```python
from build123d import *

# Parameters (mm, degrees)
BOSS_EXTRUDE1_DEPTH = 2.54
BOSS_EXTRUDE2_DEPTH = 2.54
BOSS_EXTRUDE3_DEPTH = 2.54
SKETCH6_W           = 2.54
SKETCH6_H           = 76.2
BOSS_EXTRUDE4_DEPTH = 76.2
CUT_EXTRUDE1_REACH  = 133.982
SKETCH8_W           = 2.54
SKETCH8_H           = 78.74
BOSS_EXTRUDE5_DEPTH = 76.2
CUT_EXTRUDE2_REACH  = 133.982
SKETCH10_W          = 78.74
SKETCH10_H          = 2.54
BOSS_EXTRUDE6_DEPTH = 76.2
CUT_EXTRUDE3_REACH  = 133.982
CUT_EXTRUDE5_DEPTH  = 132.982271537
CUT_EXTRUDE6_DEPTH  = 132.982271537
CUT_EXTRUDE9_DEPTH  = 76.2
BOSS_EXTRUDE7_DEPTH = 7.62
BOSS_EXTRUDE8_DEPTH = 5.08
BOSS_EXTRUDE9_DEPTH = 5.08
SKETCH34_R          = 2
CUT_EXTRUDE11_DEPTH = 12.7
SKETCH35_R          = 2
CUT_EXTRUDE13_DEPTH = 12.7
SKETCH36_R          = 2
CUT_EXTRUDE14_DEPTH = 12.7


with BuildPart() as part:
    # Sketch1 → Boss-Extrude1 (new body)
    with BuildSketch(Plane.XY):
        Polygon((0, 76.2), (0, 0), (76.2, 0), (76.2, 25.4), (25.4, 76.2), align=None)
    extrude(amount=BOSS_EXTRUDE1_DEPTH)

    # Sketch3 → Boss-Extrude2 (add)
    with BuildSketch(Plane.ZY):
        Polygon((0, 76.2), (25.4, 76.2), (76.2, 25.4), (76.2, 0), (0, 0), align=None)
    extrude(amount=BOSS_EXTRUDE2_DEPTH)

    # Sketch5 → Boss-Extrude3 (add)
    with BuildSketch(Plane.XZ):
        Polygon((-2.54, 76.2), (-2.54, 0), (76.2, 0), (76.2, 25.4), (22.86, 76.2), align=None)
    extrude(amount=BOSS_EXTRUDE3_DEPTH)

    # Sketch6 → Boss-Extrude4 (add)
    with BuildSketch(Plane.XY):
        with Locations((3.81, 38.1)):
            Rectangle(SKETCH6_W, SKETCH6_H)
    extrude(amount=BOSS_EXTRUDE4_DEPTH)

    # Sketch7 → Cut-Extrude1 (cut, up to next)
    with BuildSketch(Plane(origin=(0, 0, 0), x_dir=(0, 0, -1), z_dir=(1, 0, 0)), mode=Mode.PRIVATE) as cut_extrude1_sk1:
        Polygon((-25.4, 76.2), (-76.2, 25.4), (-76.2, 76.2), align=None)
    cut_extrude1_tool1 = extrude(cut_extrude1_sk1.sketch, amount=CUT_EXTRUDE1_REACH, mode=Mode.PRIVATE) & part.part
    add(cut_extrude1_tool1.solids().sort_by_distance((0, 59.266667, 59.266667))[0], mode=Mode.SUBTRACT)

    # Sketch8 → Boss-Extrude5 (add)
    with BuildSketch(Plane(origin=(0, 0, 0), x_dir=(0, 0, -1), z_dir=(1, 0, 0))):
        with Locations((-6.35, 36.83)):
            Rectangle(SKETCH8_W, SKETCH8_H)
    extrude(amount=BOSS_EXTRUDE5_DEPTH)

    # Sketch9 → Cut-Extrude2 (cut, up to next)
    with BuildSketch(Plane.XY, mode=Mode.PRIVATE) as cut_extrude2_sk1:
        Polygon((76.2, 25.4), (25.4, 76.2), (76.2, 76.2), align=None)
    cut_extrude2_tool1 = extrude(cut_extrude2_sk1.sketch, amount=CUT_EXTRUDE2_REACH, mode=Mode.PRIVATE) & part.part
    add(cut_extrude2_tool1.solids().sort_by_distance((59.266667, 59.266667, 0))[0], mode=Mode.SUBTRACT)

    # Sketch10 → Boss-Extrude6 (add)
    with BuildSketch(Plane.XY):
        with Locations((36.83, 3.81)):
            Rectangle(SKETCH10_W, SKETCH10_H)
    extrude(amount=BOSS_EXTRUDE6_DEPTH)

    # Sketch11 → Cut-Extrude3 (cut, up to next)
    with BuildSketch(Plane(origin=(0, 0, 0), x_dir=(1, 0, 0), z_dir=(0, 1, 0)), mode=Mode.PRIVATE) as cut_extrude3_sk1:
        Polygon((22.86, -76.2), (76.2, -25.4), (76.2, -76.2), align=None)
    cut_extrude3_tool1 = extrude(cut_extrude3_sk1.sketch, amount=CUT_EXTRUDE3_REACH, mode=Mode.PRIVATE) & part.part
    add(cut_extrude3_tool1.solids().sort_by_distance((58.42, 0, 59.266667))[0], mode=Mode.SUBTRACT)

    # Sketch12 → Cut-Extrude5 (cut, through all)
    with BuildSketch(Plane(origin=(0, 0, 0), x_dir=(0, 0, -1), z_dir=(1, 0, 0))):
        Polygon((-5.08, 5.08), (-5.08, 2.54), (-7.62, 2.54), (-7.62, 0), (-2.54, 0), (-2.54, 5.08), align=None)
    extrude(amount=CUT_EXTRUDE5_DEPTH, mode=Mode.SUBTRACT)

    # Sketch13 → Cut-Extrude6 (cut, through all)
    with BuildSketch(Plane(origin=(0, 0, 0), x_dir=(1, 0, 0), z_dir=(0, 1, 0))):
        Polygon((0, -2.54), (0, -7.62), (2.54, -7.62), (2.54, -5.08), (5.08, -5.08), (5.08, -2.54), align=None)
    extrude(amount=CUT_EXTRUDE6_DEPTH, mode=Mode.SUBTRACT)

    # Sketch15 → Cut-Extrude9 (cut)
    with BuildSketch(Plane.XY.offset(2.54)):
        Polygon((2.54, 5.08), (0, 5.08), (0, 0), (5.08, 0), (5.08, 2.54), (2.54, 2.54), align=None)
    extrude(amount=CUT_EXTRUDE9_DEPTH, mode=Mode.SUBTRACT)


with BuildPart() as cut_extrude9_piece_1:
    # of the separate pieces the step leaves, piece 1, a body of its own (cut_extrude9_pieces)
    add(part.part.solids().sort_by_distance((0, 0, 2.54))[0])



with BuildPart() as cut_extrude9_piece_2:
    # of the separate pieces the step leaves, piece 2, a body of its own (cut_extrude9_pieces)
    add(part.part.solids().sort_by_distance((2.54, 2.54, 76.2))[0])


with BuildPart() as cut_extrude9_piece_1_1:
    add(cut_extrude9_piece_1.part)

    add(cut_extrude9_piece_2.part)  # Boss-Extrude7 merges Cut-Extrude9 piece 2
    # Sketch17 → Boss-Extrude7 (add)
    with BuildSketch(Plane(origin=(0, 0, 0), x_dir=(-1, 0, 0), z_dir=(0, 0, -1))):
        Polygon((-67.219743879, 34.380256121), (-34.380256121, 67.219743879), (-30.788153673, 63.627641431), (-63.627641431, 30.788153673), align=None)
    extrude(amount=-BOSS_EXTRUDE7_DEPTH)

    # Sketch18 → Boss-Extrude8 (add)
    with BuildSketch(Plane(origin=(0, 0, 0), x_dir=(1, 0, 0), z_dir=(0, 1, 0))):
        Polygon((32.056551724, -67.44137931), (67.003448276, -34.15862069), (63.5, -30.48), (28.553103448, -63.762758621), align=None)
    extrude(amount=BOSS_EXTRUDE8_DEPTH)

    # Sketch19 → Boss-Extrude9 (add)
    with BuildSketch(Plane(origin=(0, 0, 0), x_dir=(0, 0, -1), z_dir=(1, 0, 0))):
        Polygon((-32.545001849, 69.054998151), (-67.219743879, 34.380256121), (-63.627641431, 30.788153673), (-28.9528994, 65.462895703), align=None)
    extrude(amount=BOSS_EXTRUDE9_DEPTH)

    # Sketch34 → Cut-Extrude11 (cut, symmetric)
    with BuildSketch(Plane(origin=(0, 0, 0), x_dir=(0, 0, -1), z_dir=(1, 0, 0))):
        with Locations((-15.24, 57.15)):
            Circle(SKETCH34_R)
        with Locations((-15.24, 29.21)):
            Circle(SKETCH34_R)
        with Locations((-31.75, 12.7)):
            Circle(SKETCH34_R)
        with Locations((-57.15, 12.7)):
            Circle(SKETCH34_R)
    extrude(amount=CUT_EXTRUDE11_DEPTH, both=True, mode=Mode.SUBTRACT)

    # Sketch35 → Cut-Extrude13 (cut, symmetric)
    with BuildSketch(Plane(origin=(0, 0, 0), x_dir=(1, 0, 0), z_dir=(0, 1, 0))):
        with Locations(Location((12.7, -57.15, 0), (0, 0, 270))):
            Circle(SKETCH35_R)
        with Locations(Location((12.7, -31.75, 0), (0, 0, 270))):
            Circle(SKETCH35_R)
        with Locations(Location((29.21, -15.24, 0), (0, 0, 270))):
            Circle(SKETCH35_R)
        with Locations(Location((57.15, -15.24, 0), (0, 0, 270))):
            Circle(SKETCH35_R)
    extrude(amount=CUT_EXTRUDE13_DEPTH, both=True, mode=Mode.SUBTRACT)

    # Sketch36 → Cut-Extrude14 (cut, symmetric)
    with BuildSketch(Plane.XY):
        with Locations((57.15, 12.7)):
            Circle(SKETCH36_R)
        with Locations((29.21, 12.7)):
            Circle(SKETCH36_R)
        with Locations((12.7, 29.21)):
            Circle(SKETCH36_R)
        with Locations((12.7, 57.15)):
            Circle(SKETCH36_R)
    extrude(amount=CUT_EXTRUDE14_DEPTH, both=True, mode=Mode.SUBTRACT)


solid = cut_extrude9_piece_1_1.part
```
The listing builds one solid part. Answer for the finished solid, in the listing's coordinates (mm). A direction names the side the tool comes from. Coordinates: 2 decimals unless noted, no trailing zeros. Order: outer loops, then holes, each group sorted by start corner. A loop starts at its lowest first (then second) coordinate and runs counter-clockwise, first axis right, second up. Notation, with made-up numbers: M 39.25,23 L 98.25,23 A26 cw 98.25,39 Z; hole C 79.5,28 d8. An arc over 180 degrees is marked long. Answer as a JSON object with one key per item and string values. Group by question number.
1. Section A-A on z = 24 is taken. Write down the section's boundary in (x, y), then the cut area to 3 significant figures.
2. Straight lines are drawn through the part: line 1 (Y direction, x = 4, z = 15); line 2 (Y direction, x = 43, z = 12); line 3 (Z direction, x = 31.5, y = 33.5). For each, find the intervals that lie inside material, in ascending order.
3. Section B-B on y = 20 is taken. Write down the section's boundary in (x, z).
4. A tool of negligible diameter and unlimited length cuts with its end or side. For faces 5 (the flat face through (32, 33, 7.62)), 6 (the cylindrical face through (11.934, -1.252, 33.597)), 7 (the flat face through (46.27, 1.25, 46.89)), from which of +Z, -Z, +X, -X, +Y, -Y can it reach the whole face along a straight path? Write none if from no direction.
5. Section D-D on z = 57.5 is taken. Write down the section's boundary in (x, y) (3 decimals).
6. Section C-C on x = 60.5 is taken. Write down the section's boundary in (y, z).
7. Determine the mould class of faces 1 (the cylindrical face through (11.934, 3.792, 58.997)), 2 (the flat face through (30.28, 1.252, 65.576)), 3 (the flat face through (65.4, 32.56, 3.79)), 4 (the flat face through (9, 76.2, 7)) for opening direction X: released by +X, released by -X, zero draft, split by the parting line, or undercut.
8. Flat-ended cylindrical pins translate along their axes: P1, Ø2.5, axis at x = 57.15, z = 15.24, coming from the -Y side; P2, Ø6.5, axis at y = 57.15, z = 15.24, coming from the +X side; P3, Ø8, axis at x = 37, y = 50, coming from the +Z side; P4, Ø4.5, axis at x = 12.7, z = 31.75, coming from the +Y side. Find the tip coordinate at first contact, or state that the pin passes through.
Values follow:
{
 "1": {"outline": "M -2.54,-2.54 L 76.2,-2.54 L 76.2,0 L 0,0 L 0,76.2 L -2.54,76.2 Z; M 2.54,2.54 L 76.2,2.54 L 76.2,5.08 L 5.08,5.08 L 5.08,76.2 L 2.54,76.2 Z", "area": "761 mm2"},
 "2": {"line 1": "-2.54 to 0, 2.54 to 27.22, 31.2 to 55.16, 59.14 to 76.2", "line 2": "-2.54 to 0, 2.54 to 5.08", "line 3": "0 to 2.54, 5.08 to 7.62"},
 "3": {"outline": "M -2.54,0 L 76.2,0 L 76.2,2.54 L 0,2.54 L 0,76.2 L -2.54,76.2 Z; M 2.54,5.08 L 76.2,5.08 L 76.2,7.62 L 5.08,7.62 L 5.08,76.2 L 2.54,76.2 Z"},
 "4": {"face 5": "+Z, +X, +Y", "face 6": "+Y, -Y", "face 7": "none"},
 "5": {"outline": "M -2.54,-2.54 L 10.731,-2.54 L 10.731,0 L 0,0 L 0,10.731 L -2.54,10.731 Z; M -2.54,14.669 L 0,14.669 L 0,36.916 L 2.54,36.916 L 2.54,14.669 L 5.08,14.669 L 5.08,44.1 L -2.54,44.1 Z; M 2.54,2.54 L 10.731,2.54 L 10.731,5.08 L 5.08,5.08 L 5.08,10.731 L 2.54,10.731 Z; M 14.669,-2.54 L 42.495,-2.54 L 42.495,5.08 L 14.669,5.08 L 14.669,2.54 L 35.129,2.54 L 35.129,0 L 14.669,0 Z"},
 "6": {"outline": "M -2.54,0 L 41.1,0 L 41.1,7.62 L 5.08,7.62 L 5.08,40.35 L -2.54,40.35 Z; hole M 0,2.54 L 33.92,2.54 L 33.92,5.08 L 2.54,5.08 L 2.54,33.34 L 0,33.34 Z"},
 "7": {"face 1": "undercut", "face 2": "undercut", "face 3": "released by +X", "face 4": "zero draft"},
 "8": {"P1": "through", "P2": "x = 5.08", "P3": "z = 7.62", "P4": "y = 5.08"}
}
